from build123d import *

# Parameters (mm, degrees)
SKETCH1_W             = 6
SKETCH1_H             = 10.9
BOSS_EXTRUDE1_DEPTH   = 3
BOSS_EXTRUDE1_2_DEPTH = 3
SKETCH2_W             = 25.1
SKETCH2_H             = 10.9
BOSS_EXTRUDE2_DEPTH   = 1.9


with BuildPart() as part:
    # Sketch1 → Boss-Extrude1 (new body)
    with BuildSketch(Plane(origin=(0, 0, 0), x_dir=(1, 0, 0), z_dir=(0, 1, 0))):
        with Locations((-8, 0)):
            Rectangle(SKETCH1_W, SKETCH1_H)
    extrude(amount=BOSS_EXTRUDE1_DEPTH)



with BuildPart() as body_2:
    # Sketch1 → Boss-Extrude1 2 (new body)
    with BuildSketch(Plane(origin=(0, 0, 0), x_dir=(1, 0, 0), z_dir=(0, 1, 0))):
        with Locations((8, 0)):
            Rectangle(SKETCH1_W, SKETCH1_H)
    extrude(amount=BOSS_EXTRUDE1_2_DEPTH)


with BuildPart() as part_1:
    add(part.part)

    add(body_2.part)  # Boss-Extrude2 merges body 2
    # Sketch2 → Boss-Extrude2 (add)
    with BuildSketch(Plane(origin=(0, 3, 0), x_dir=(1, 0, 0), z_dir=(0, 1, 0))):
        Rectangle(SKETCH2_W, SKETCH2_H)
    extrude(amount=BOSS_EXTRUDE2_DEPTH)


solid = part_1.part
Input: part model. Units: mm. Frame: model coordinates. A direction names the side the tool comes from. Round coordinates to 2 decimals unless told otherwise and drop trailing zeros. Write each loop counter-clockwise with the first axis right and the second up, starting at its lowest first coordinate (ties: lowest second). Pieces come first, ordered by that corner, then holes.
1) Cut plane B-B (z = -3.25). Return the cut outline in (x, y).
2) Ray query, L1, parallel to X at y = 2.2, z = -2; L2, parallel to Y at x = 3, z = -4.75. Return the intervals inside material, ascending.
3) Contact query for flat-ended pins moving along their axis: P1, Ø2.5, axis at y = 2, z = -2, coming from the -X side; P2, Ø0.5, axis at x = -12, z = 1, coming from the -Y side; P3, Ø1.5, axis at y = 2, z = 1, coming from the +X side; P4, Ø1.5, axis at y = 1, z = -2.5, coming from the -X side. Output: stop coordinate, or through.
4) Cut plane A-A (y = 0.45). Return the cut outline in (x, z), then the cut area to 3 significant figures.
5) Reachability of faces 1 (the flat face through (12, 3, 0)), 2 (the flat face through (0, 4, -5.45)), 3 (the flat face through (5, 1, 0)), 4 (the flat face through (-11, 1, 0)) from +Z, -Z, +X, -X, +Y, -Y: full face, straight path, thin tool, end or side. Return the list, or none.
6) Cut plane C-C (x = -2.5). Return the cut outline in (y, z), then the cut area to 3 significant figures.
7) Draft query along X for faces 5 (the flat face through (-5, 1, 0)), 6 (the flat face through (11, 1, 0)), 7 (the flat face through (0, 3, 0)), 8 (the flat face through (8, 0, 0)). Return one class per face: pulls with the +X half, pulls with the -X half, needs draft (parallel to the pull), parting line crosses it, or undercut.
Geometry says:
1. outline: (-12.55, 3) - (-11, 3) - (-11, 0) - (-5, 0) - (-5, 3) - (5, 3) - (5, 0) - (11, 0) - (11, 3) - (12.55, 3) - (12.55, 4.9) - (-12.55, 4.9) - close
2. L1: x = -11 to -5, 5 to 11
2. L2: y = 3 to 4.9
3. P1: stops at x = -12.55
3. P2: stops at y = 3
3. P3: stops at x = 11
3. P4: stops at x = -11
4. outline: (-11, -5.45) - (-5, -5.45) - (-5, 5.45) - (-11, 5.45) - close; (5, -5.45) - (11, -5.45) - (11, 5.45) - (5, 5.45) - close
4. area: 131 mm2
5. face 1: +Z, -Z, +X, -Y
5. face 2: -Z, +X, -X, +Y, -Y
5. face 3: +Z, -Z, -Y
5. face 4: +Z, -Z, -X, -Y
6. outline: (3, -5.45) - (4.9, -5.45) - (4.9, 5.45) - (3, 5.45) - close
6. area: 20.7 mm2
7. face 5: undercut
7. face 6: pulls with the +X half
7. face 7: undercut
7. face 8: needs draft
